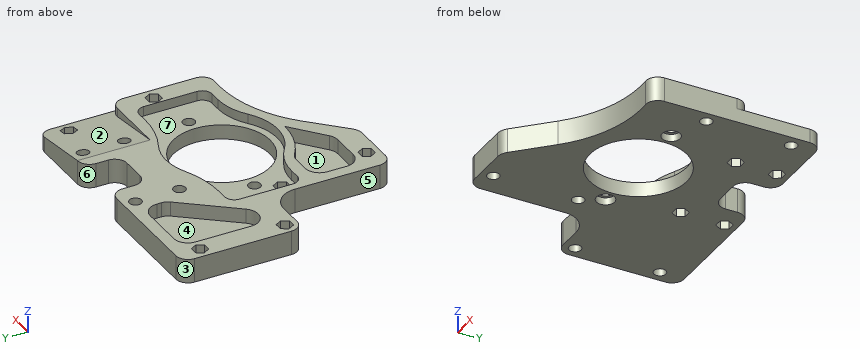
from build123d import *

# Parameters (mm, degrees)
FIGURE_EXTRUDE_DEPTH      = 10
SKETCH2_R                 = 20
SKETCH2_R_2               = 2.5
ALL_5MM_HOLES_DEPTH       = 11
ANGLED_PLANE_CUT_DEPTH    = 30
ANGLED_PLANE_FILLET_R     = 5
TRIANGULAR_CUT_DEPTH      = 6
MIDDLE_CIRCULAR_CUT_DEPTH = 4
CUT_EXTRUDE12_DEPTH       = 6
SKETCH7_R                 = 3.75
CUT_EXTRUDE13_DEPTH       = 3
CUT_EXTRUDE14_DEPTH       = 5
CUT_EXTRUDE15_DEPTH       = 7
CUT_EXTRUDE17_DEPTH       = 7


with BuildPart() as part:
    # Sketch1 → Figure Extrude (new body)
    with BuildSketch(Plane.XY):
        with BuildLine():
            Line((0, 30), (-45, 30))
            ThreePointArc((-45, 30), (-48.535533906, 28.535533906), (-50, 25))
            Line((-50, 25), (-50, -15))
            ThreePointArc((-50, -15), (-48.535533906, -18.535533906), (-45, -20))
            Line((-45, -20), (-35, -20))
            ThreePointArc((-35, -20), (-27.928932188, -22.928932188), (-25, -30))
            Line((-25, -30), (-25, -65))
            ThreePointArc((-25, -65), (-23.535533906, -68.535533906), (-20, -70))
            Line((-20, -70), (-2.48528, -70))
            ThreePointArc((-2.48528, -70), (-0.189179406, -69.543277195), (1.757360687, -68.242640687))
            Line((1.757360687, -68.242640687), (15.280716751, -54.719284623))
            ThreePointArc((15.280716751, -54.719284623), (33.367897146, -43.085414566), (54.651065241, -40))
            ThreePointArc((54.651065241, -40), (58.409935938, -38.669011007), (60, -35.012190407))
            Line((60, -35.012190407), (60, 25))
            ThreePointArc((60, 25), (58.535533906, 28.535533906), (55, 30))
            Line((55, 30), (30, 30))
            ThreePointArc((30, 30), (26.464466094, 28.535533906), (25, 25))
            Line((25, 25), (25, 20))
            ThreePointArc((25, 20), (23.535533906, 16.464466094), (20, 15))
            Line((20, 15), (10, 15))
            ThreePointArc((10, 15), (6.464466094, 16.464466094), (5, 20))
            Line((5, 20), (5, 25))
            ThreePointArc((5, 25), (3.535533906, 28.535533906), (0, 30))
        make_face()
    extrude(amount=FIGURE_EXTRUDE_DEPTH)

    # Sketch2 → All 5mm Holes (cut, through all)
    with BuildSketch(Plane.XY):
        with Locations((15, -21.4)):
            Circle(SKETCH2_R)
        with Locations((55, 20)):
            Circle(SKETCH2_R_2)
        with Locations((55, -15)):
            Circle(SKETCH2_R_2)
        with Locations((-45, 20)):
            Circle(SKETCH2_R_2)
        with Locations((-45, -15)):
            Circle(SKETCH2_R_2)
        with Locations((35, 25)):
            Circle(SKETCH2_R_2)
        with Locations((35, 7.98621)):
            Circle(SKETCH2_R_2)
        with Locations((-5, 25)):
            Circle(SKETCH2_R_2)
        with Locations((-5, 6.85613)):
            Circle(SKETCH2_R_2)
        with Locations((-15, -30)):
            Circle(SKETCH2_R_2)
        with Locations((-15, -65)):
            Circle(SKETCH2_R_2)
        with Locations((-10, -21.4)):
            Circle(SKETCH2_R_2)
        with Locations((40, -21.4)):
            Circle(SKETCH2_R_2)
    extrude(amount=ALL_5MM_HOLES_DEPTH, mode=Mode.SUBTRACT)

    # Sketch3 → Angled Plane Cut (cut)
    with BuildSketch(Plane(origin=(0, 30, 0), x_dir=(1, 0, 0), z_dir=(0, 1, 0))):
        Polygon((30, -10), (60, -5.714340401), (60, -10), align=None)
    extrude(amount=-ANGLED_PLANE_CUT_DEPTH, mode=Mode.SUBTRACT)

    # Angled Plane Fillet
    angled_plane_fillet_edges = [part.edges().sort_by_distance(p)[0] for p in [
        (60, 0, 7.8571702),
    ]]
    fillet(angled_plane_fillet_edges, radius=ANGLED_PLANE_FILLET_R)

    # Sketch4 → Triangular cut (cut)
    with BuildSketch(Plane.XY.offset(10)):
        with BuildLine():
            Line((-34.217521015, 25), (-16.217521015, 25))
            ThreePointArc((-16.217521015, 25), (-11.974880328, 23.242640687), (-10.217521015, 19))
            Line((-10.217521015, 19), (-10.217521015, 17.10468))
            ThreePointArc((-10.217521015, 17.10468), (-10.499794454, 15.447216646), (-11.31479, 13.976623119))
            Line((-11.31479, 13.976623119), (-28.69474373, -7.74817))
            ThreePointArc((-28.69474373, -7.74817), (-35.753124005, -9.772794597), (-40, -3.782478985))
            Line((-40, -3.782478985), (-40, 19.217521015))
            ThreePointArc((-40, 19.217521015), (-38.306351117, 23.306351117), (-34.217521015, 25))
        make_face()
    extrude(amount=-TRIANGULAR_CUT_DEPTH, mode=Mode.SUBTRACT)

    # Sketch5 → Middle Circular Cut (cut)
    with BuildSketch(Plane.XY.offset(10)):
        with BuildLine():
            Line((-21.5, -9), (-21.5, -31))
            ThreePointArc((-21.5, -31), (-20.328427125, -33.828427125), (-17.5, -35))
            Line((-17.5, -35), (-13, -35))
            ThreePointArc((-13, -35), (-5.552074466, -36.216817559), (1.121326058, -39.740730891))
            ThreePointArc((1.121326058, -39.740730891), (15, -44.4), (28.878673942, -39.740730891))
            ThreePointArc((28.878673942, -39.740730891), (35.552074466, -36.216817559), (43, -35))
            Line((43, -35), (47.5, -35))
            ThreePointArc((47.5, -35), (50.328427125, -33.828427125), (51.5, -31))
            Line((51.5, -31), (51.5, -9))
            ThreePointArc((51.5, -9), (50.328427125, -6.171572875), (47.5, -5))
            Line((47.5, -5), (43, -5))
            ThreePointArc((43, -5), (33.893145617, -3.941200412), (25.272125284, -0.821286674))
            ThreePointArc((25.272125284, -0.821286674), (15, 1.6), (4.727874716, -0.821286674))
            ThreePointArc((4.727874716, -0.821286674), (-3.893145617, -3.941200412), (-13, -5))
            Line((-13, -5), (-17.5, -5))
            ThreePointArc((-17.5, -5), (-20.328427125, -6.171572875), (-21.5, -9))
        make_face()
    extrude(amount=-MIDDLE_CIRCULAR_CUT_DEPTH, mode=Mode.SUBTRACT)

    # Sketch6 → Cut-Extrude12 (cut)
    with BuildSketch(Plane.XY.offset(10)):
        with BuildLine():
            Line((-20, -54), (-20, -46.1088))
            ThreePointArc((-20, -46.1088), (-18.242640687, -41.866159313), (-14, -40.1088))
            Line((-14, -40.1088), (-7.34446, -40.1088))
            ThreePointArc((-7.34446, -40.1088), (-5.468840073, -40.409497421), (-3.781218172, -41.281450036))
            ThreePointArc((-3.781218172, -41.281450036), (5.113938727, -45.877358228), (15, -47.462281209))
            Line((15, -47.462281209), (1.587090544, -58.613720541))
            ThreePointArc((1.587090544, -58.613720541), (-0.209415261, -59.642797323), (-2.24873828, -60))
            Line((-2.24873828, -60), (-14, -60))
            ThreePointArc((-14, -60), (-18.242640687, -58.242640687), (-20, -54))
        make_face()
    extrude(amount=-CUT_EXTRUDE12_DEPTH, mode=Mode.SUBTRACT)

    # Sketch7 → Cut-Extrude13 (cut)
    with BuildSketch(Plane(origin=(0, 0, 0), x_dir=(-1, 0, 0), z_dir=(0, 0, -1))):
        with Locations((-40, -21.4)):
            Circle(SKETCH7_R)
        with Locations((10, -21.4)):
            Circle(SKETCH7_R)
    extrude(amount=-CUT_EXTRUDE13_DEPTH, mode=Mode.SUBTRACT)

    # Sketch8 → Cut-Extrude14 (cut)
    with BuildSketch(Plane(origin=(0, 0, 0), x_dir=(-1, 0, 0), z_dir=(0, 0, -1))):
        Polygon((-33.41229, 27.749994388), (-36.58771, 27.749994388), (-38.17542, 25), (-36.58771, 22.250005612), (-33.41229, 22.250005612), (-31.82458, 25), align=None)
        Polygon((-33.41229, 10.736204388), (-36.58771, 10.736204388), (-38.17542, 7.98621), (-36.58771, 5.236215612), (-33.41229, 5.236215612), (-31.82458, 7.98621), align=None)
        Polygon((3.41229, 9.606124388), (1.82458, 6.85613), (3.41229, 4.106135612), (6.58771, 4.106135612), (8.17542, 6.85613), (6.58771, 9.606124388), align=None)
        Polygon((3.41229, 27.749994388), (1.82458, 25), (3.41229, 22.250005612), (6.58771, 22.250005612), (8.17542, 25), (6.58771, 27.749994388), align=None)
    extrude(amount=-CUT_EXTRUDE14_DEPTH, mode=Mode.SUBTRACT)

    # Sketch9 → Cut-Extrude15 (cut)
    with BuildSketch(Plane.XY.offset(10)):
        Polygon((-41.82458, 20), (-43.41229, 22.749994388), (-46.58771, 22.749994388), (-48.17542, 20), (-46.58771, 17.250005612), (-43.41229, 17.250005612), align=None)
        Polygon((-43.41229, -17.749994388), (-41.82458, -15), (-43.41229, -12.250005612), (-46.58771, -12.250005612), (-48.17542, -15), (-46.58771, -17.749994388), align=None)
        Polygon((-13.41229, -67.749994388), (-11.82458, -65), (-13.41229, -62.250005612), (-16.58771, -62.250005612), (-18.17542, -65), (-16.58771, -67.749994388), align=None)
        Polygon((56.58771, -17.749994388), (58.17542, -15), (56.58771, -12.250005612), (53.41229, -12.250005612), (51.82458, -15), (53.41229, -17.749994388), align=None)
        Polygon((56.58771, 17.250005612), (58.17542, 20), (56.58771, 22.749994388), (53.41229, 22.749994388), (51.82458, 20), (53.41229, 17.250005612), align=None)
    extrude(amount=-CUT_EXTRUDE15_DEPTH, mode=Mode.SUBTRACT)

    # Sketch9_4 → Cut-Extrude17 (cut)
    with BuildSketch(Plane.XY.offset(10)):
        Polygon((-13.41229, -32.749994388), (-11.82458, -30), (-13.41229, -27.250005612), (-16.58771, -27.250005612), (-18.17542, -30), (-16.58771, -32.749994388), align=None)
    extrude(amount=-CUT_EXTRUDE17_DEPTH, mode=Mode.SUBTRACT)


solid = part.part
Read the model definition and answer for the solid it produces. Units are mm, in the model's axes. Face numbers are marked on the shaded views. A direction names the side the tool comes from. Give positions to 0.01 mm unless a question says otherwise; leave off trailing zeros. Write each loop counter-clockwise with the first axis right and the second up, starting at its lowest first coordinate (ties: lowest second). Pieces come first, ordered by that corner, then holes. Notation, with made-up numbers: (30.5, 80) - (58.5, 80) arc R6 ccw to (58.5, 88) - close; hole circle Ø9 at (-12, 56). An arc over 180 degrees is marked (long way). Answer in a Markdown table with one row per item. Add a question column.
Item 1: Section B-B, the plane x = -37.5 is taken. Write down the section's boundary in (y, z), and give its area (3 significant figures).
Item 2: Section C-C, the plane x = 27.5 is taken. Write down the section's boundary in (y, z).
Item 3: Determine the mould class of the marked faces 1, 2, 3 and 4 for opening direction X: pulls with the +X half, pulls with the -X half, needs draft (parallel to the pull), parting line crosses it, or undercut.
Item 4: Section A-A, the plane x = 41 is taken. Write down the section's boundary in (y, z).
Item 5: Flat-ended cylindrical pins translate along their axes: P1, Ø3, axis at x = -25, z = 5.5, coming from the -Y side; P2, Ø6, axis at x = 11.5, z = 7.5, coming from the +Y side; P3, Ø12, axis at x = 34, y = -18, coming from the +Z side. Find the tip coordinate at first contact, or state that the pin passes through.
Item 6: A tool of negligible diameter and unlimited length cuts with its end or side. For the marked faces 5, 6 and 7, from which of +Z, -Z, +X, -X, +Y, -Y can it reach the whole face along a straight path? Write none if from no direction.
Item 7: Find the intervals of material crossed by L1, parallel to Y at x = -10, z = 4.2; L2, parallel to X at y = 25, z = 3.25; L3, parallel to Y at x = -44.5, z = 9.75, in increasing order.
Recorded:
| question | item | result |
|---|---|---|
| 1 | outline | (-20, 0) - (30, 0) - (30, 10) - (23.98, 10) - (23.98, 4) - (-8.83, 4) - (-8.83, 10) - (-20, 10) - close |
| 1 | area | 303 mm2 |
| 2 | outline | (-45.71, 0) - (-37.01, 0) - (-37.01, 6) - (-40.71, 6) - (-40.71, 10) - (-45.71, 10) - close; (-5.79, 0) - (29.33, 0) - (29.33, 10) - (-1.85, 10) - (-1.85, 6) - (-5.79, 6) - close |
| 3 | face 1 | undercut |
| 3 | face 2 | pulls with the +X half |
| 3 | face 3 | pulls with the -X half |
| 3 | face 4 | undercut |
| 4 | outline | (-40.9, 0) - (-25.01, 0) - (-25.01, 3) - (-23.69, 3) - (-23.69, 6) - (-35.09, 6) - (-35.09, 10) - (-40.9, 10) - close; (-19.11, 3) - (-17.79, 3) - (-17.79, 0) - (30, 0) - (30, 8.43) - (0, 8.43) - (0, 10) - (-4.95, 10) - (-4.95, 6) - (-19.11, 6) - close |
| 5 | P1 | stops at y = -68.57 |
| 5 | P2 | stops at y = 15.23 |
| 5 | P3 | stops at z = 6 |
| 6 | face 5 | +Z, -Z, -X, -Y |
| 6 | face 6 | +Z, -Z, +Y |
| 6 | face 7 | +Z |
| 7 | L1 | y = -70 to -60, -40.11 to -23.9, -18.9 to 30 |
| 7 | L2 | x = -50 to -8.18, -1.82 to 5, 25 to 31.82, 38.18 to 60 |
| 7 | L3 | y = -20 to -17.75, -12.25 to 17.25, 22.75 to 30 |
